Geometry: see drawing. Coordinates: mm, zero at the bounding-box minimum. Give positions to 0.01 mm unless a question says otherwise; leave off trailing zeros. Loops run counter-clockwise (first coordinate to the right, second up) from the corner with the lowest first, then second, coordinate; pieces in that order, holes last. Notation, with made-up numbers: (14.5, 50.25) -> (19.5, 50.25) arc R28 ccw to (19.5, 88.25) -> close; hole circle Ø2 at (31, 4). An arc over 180 degrees is marked (long way). One line per question, with ' | ' between items.
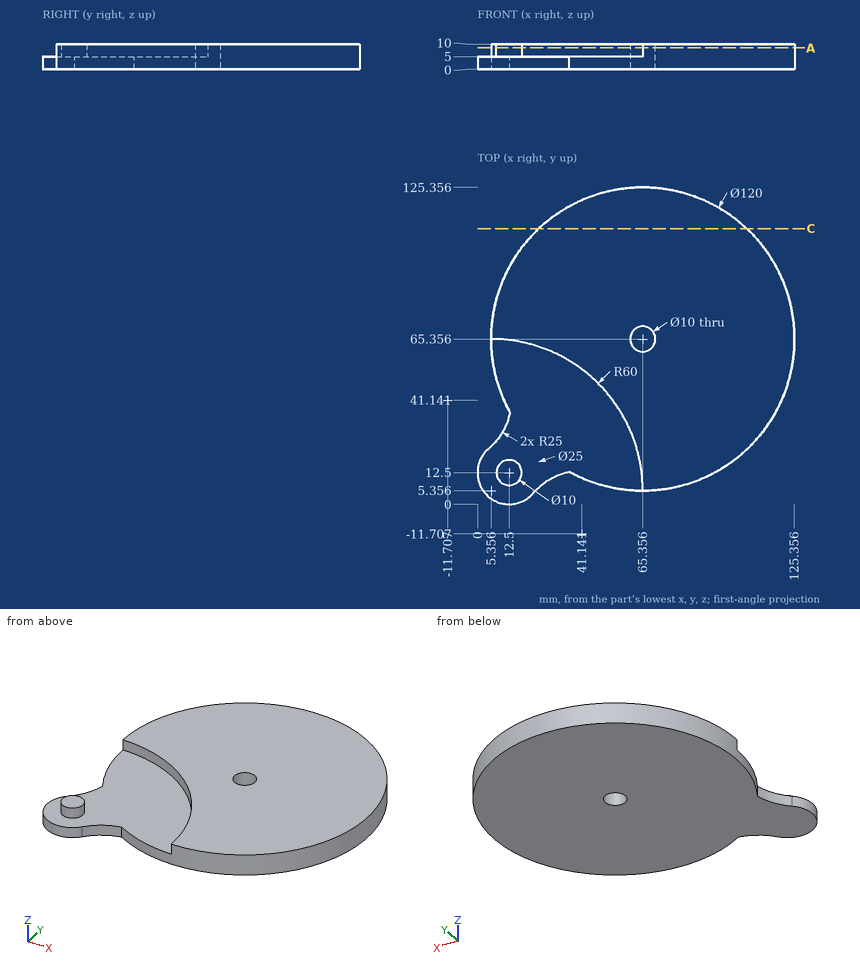
1. Ray query, line 1 along Z through (x, y) = (37, 41.5); line 2 along X through (y, z) = (59.5, 6.5) (1 decimal); line 3 along Y through (x, z) = (38, 2.25) (1 decimal). Return the intervals inside material, ascending. Write a range as from..to.
Determined:
line 1: z = 0..5 | line 2: x = 31.2..125.1 | line 3: y = 12..118.8
2. Pin query (flat end, axial travel): P1, Ø5, axis at x = 91.5, z = 4.5, coming from the -Y side; P2, Ø4, axis at x = 108, z = 7.5, coming from the -Y side; P3, Ø11.5, axis at x = 65.36, y = 65.36, coming from the +Z side; P4, Ø5, axis at x = 103, z = 8, coming from the +Y side. Return the tip coordinate at first contact, or that it passes through.
Determined:
P1: stops at y = 10.21 | P2: stops at y = 21.22 | P3: stops at z = 10 | P4: stops at y = 113.99
3. Section query C-C (y = 109). Output: boundary loops of the cut face in (x, z).
Determined:
outline: (24.18, 0) -> (106.53, 0) -> (106.53, 10) -> (24.18, 10) -> close
4. Section query A-A (z = 8.5). Output: boundary loops of the cut face in (x, y).
Determined:
outline: (5.36, 65.36) arc R60 cw to (65.36, 5.36) arc R60 ccw (long way) to start; circle Ø10 at (12.5, 12.5); hole circle Ø10 at (65.36, 65.36)
